Geometry: final body of the model. Coordinates: model frame, mm. Round coordinates to 2 decimals unless told otherwise and drop trailing zeros. Loops run counter-clockwise (first coordinate to the right, second up) from the corner with the lowest first, then second, coordinate; pieces in that order, holes last. Notation, with made-up numbers: M -8,8 L 7,8 A14 cw 7,12 Z; hole C -0.5,57 d11. An arc over 180 degrees is marked long. Return JSON: item names as keys, results as strings.
from build123d import *

# Parameters (mm, degrees)
SKETCH1_R           = 2.75
BOSS_EXTRUDE1_DEPTH = 3.2


with BuildPart() as part:
    # Sketch1 → Boss-Extrude1 (new body)
    with BuildSketch(Plane.XY):
        Polygon((-50, 75), (-47, 72), (-9, 72), (-9, 3), (-6, 0), (6, 0), (9, 3), (9, 72), (47, 72), (50, 75), (50, 87), (47, 90), (-47, 90), (-50, 87), align=None)
        with Locations((40, 81)):
            Circle(SKETCH1_R, mode=Mode.SUBTRACT)
        with Locations((0, 40)):
            Circle(SKETCH1_R, mode=Mode.SUBTRACT)
        with Locations((0, 10)):
            Circle(SKETCH1_R, mode=Mode.SUBTRACT)
        with Locations((-40, 81)):
            Circle(SKETCH1_R, mode=Mode.SUBTRACT)
    extrude(amount=-BOSS_EXTRUDE1_DEPTH)


solid = part.part
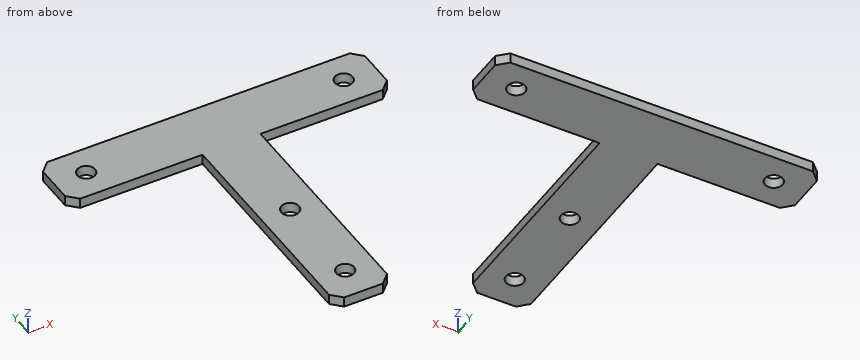
Q1. Pin query (flat end, axial travel): pin 1 (1.6 mm diameter, centred on x = -32, z = -1, fed in from -Y); pin 2 (1 mm diameter, centred on y = 32.5, z = -1, fed in from +X). Return the tip coordinate at first contact, or that it passes through.
Determined:
{"pin 1": "stops at y = 72", "pin 2": "stops at x = 9"}
Q2. Section query D-D (z = -1.35). Output: boundary loops of the cut face in (x, y).
Determined:
{"outline": "M -50,75 L -47,72 L -9,72 L -9,3 L -6,0 L 6,0 L 9,3 L 9,72 L 47,72 L 50,75 L 50,87 L 47,90 L -47,90 L -50,87 Z; hole C -40,81 d5.5; hole C 0,10 d5.5; hole C 0,40 d5.5; hole C 40,81 d5.5"}
Q3. Section query A-A (y = 40). Output: boundary loops of the cut face in (x, z), plus the area to 3 significant figures.
Determined:
{"outline": "M -9,-3.2 L -2.75,-3.2 L -2.75,0 L -9,0 Z; M 2.75,-3.2 L 9,-3.2 L 9,0 L 2.75,0 Z", "area": "40.0 mm^2"}
Q4. Section query B-B (y = 81). Output: boundary loops of the cut face in (x, z), plus the area to 3 significant figures.
Determined:
{"outline": "M -50,-3.2 L -42.75,-3.2 L -42.75,0 L -50,0 Z; M -37.25,-3.2 L 37.25,-3.2 L 37.25,0 L -37.25,0 Z; M 42.75,-3.2 L 50,-3.2 L 50,0 L 42.75,0 Z", "area": "285 mm^2"}
Q5. Section query C-C (x = -40). Output: boundary loops of the cut face in (y, z), plus the area to 3 significant figures.
Determined:
{"outline": "M 72,-3.2 L 78.25,-3.2 L 78.25,0 L 72,0 Z; M 83.75,-3.2 L 90,-3.2 L 90,0 L 83.75,0 Z", "area": "40.0 mm^2"}
Q6. Material intervals for L1, parallel to Y at x = 0, z = -0.8; L2, parallel to Y at x = -40, z = -1; L3, parallel to X at y = 21, z = -1.4, sorted ascending.
Determined:
{"L1": "y = 0 to 7.25, 12.75 to 37.25, 42.75 to 90", "L2": "y = 72 to 78.25, 83.75 to 90", "L3": "x = -9 to 9"}
